Read the model definition and answer for the solid it produces. Units are mm, in the model's axes. Give positions to 0.01 mm unless a question says otherwise; leave off trailing zeros. Loops run counter-clockwise (first coordinate to the right, second up) from the corner with the lowest first, then second, coordinate; pieces in that order, holes last. Notation, with made-up numbers: (82.25, 66.25) -> (98.25, 66.25) arc R11 ccw to (98.25, 85.25) -> close; hole circle Ø8 at (87.5, 74.5). An arc over 180 degrees is marked (long way). Return JSON: item names as keys, results as strings. Group by question number.
from build123d import *

# Parameters (mm, degrees)
BOSS_EXTRUDE1_DEPTH      = 192.925743
BOSS_EXTRUDE1_DEPTH_BACK = 146.220291
SKETCH1_R                = 7.9375
SKETCH1_R_2              = 6.4643
CUT_EXTRUDE1_DEPTH       = 331.187461377


with BuildPart() as part:
    # Sketch1 → Boss-Extrude1 (new, two sides: drawn at the far end of the back side and taken through both)
    with BuildSketch(Plane(origin=(0, 0, 0), x_dir=(0, 0, -1), z_dir=(1, 0, 0)).offset(-BOSS_EXTRUDE1_DEPTH_BACK)):
        with Locations(Location((0, 0, 0), (0, 0, 180))):
            Circle(SKETCH1_R)
        with Locations(Location((0, 0, 0), (0, 0, 180))):
            Circle(SKETCH1_R_2, mode=Mode.SUBTRACT)
    extrude(amount=BOSS_EXTRUDE1_DEPTH + BOSS_EXTRUDE1_DEPTH_BACK)

    # Sketch2 → Cut-Extrude1 (cut, through all)
    with BuildSketch(Plane(origin=(179.090362215, 7.9375, -46.327801352), x_dir=(0.11485518524691138, 0, -0.9933822458761269), z_dir=(0, 1, 0))):
        with BuildLine():
            Line((-86.538819377, 317.472174359), (-82.162836819, 279.624310791))
            ThreePointArc((-82.162836819, 279.624310791), (-81.572017256, 278.562611401), (-80.403509897, 278.229649083))
            Line((-80.403509897, 278.229649083), (-77.249521267, 278.594314296))
            ThreePointArc((-77.249521267, 278.594314296), (-76.187821877, 279.185133859), (-75.854859558, 280.353641218))
            Line((-75.854859558, 280.353641218), (-80.230842116, 318.201504786))
            Line((-80.230842116, 318.201504786), (-86.538819377, 317.472174359))
        make_face()
    extrude(amount=-CUT_EXTRUDE1_DEPTH, mode=Mode.SUBTRACT)


solid = part.part
1. Section A-A on y = 0 is taken. Determine the outline of the cut face in (x, z).
2. Section B-B on x = -116.5 is taken. Determine the outline of the cut face in (y, z) (1 decimal), then the cut area to 3 significant figures.
3. Determine the mould class of faces 1 (the cylindrical face through (20.98, -6.41, -0.84)), 2 (the cylindrical face through (20.979, -2.384, 7.571)), 3 (the flat face through (192.926, 0, -7)) for opening direction Y: pulls with the +Y half, pulls with the -Y half, needs draft (parallel to the pull), parting line crosses it, or undercut.
4. Section C-C on x = 71 is taken. Determine the outline of the cut face in (y, z) (1 decimal).
5. Straight lines are drawn through the part: line 1 (Z direction, x = 152, y = -1.5); line 2 (Y direction, x = 31, z = 0.25). For each, find the intervals that lie inside material, in ascending order. Write a range as from..to.
6. Flat-ended cylindrical pins translate along their axes: pin 1 Ø1.3 at (x, y) = (-126, 6) entering from -Z; pin 2 Ø1.5 at (x, y) = (31.5, -3) entering from +Z; pin 3 Ø3 at (x, y) = (150, 4.5) entering from -Z. Find the tip coordinate at first contact, or state that the pin passes through.
Completed:
{
 "1": {"outline": "(-146.22, -7.94) -> (192.93, -7.94) -> (192.93, -6.46) -> (-146.22, -6.46) -> close; (-146.22, 6.46) -> (192.93, 6.46) -> (192.93, 7.94) -> (-146.22, 7.94) -> close"},
 "2": {"outline": "(-7.3, -3.2) arc R7.9 ccw to (7.3, -3.2) -> (5.6, -3.2) arc R6.5 cw to (-5.6, -3.2) -> close; (-7.3, 3.2) -> (-5.6, 3.2) arc R6.5 cw to (5.6, 3.2) -> (7.3, 3.2) arc R7.9 ccw to start", "area": "47.3 mm²"},
 "3": {"face 1": "undercut", "face 2": "parting line crosses it", "face 3": "needs draft"},
 "4": {"outline": "circle Ø15.9 at (0, 0); hole circle Ø12.9 at (0, 0)"},
 "5": {"line 1": "z = -7.79..-6.29, 6.29..7.79", "line 2": "y = -7.93..-6.46, 6.46..7.93"},
 "6": {"pin 1": "stops at z = -5.86", "pin 2": "stops at z = 7.61", "pin 3": "stops at z = -7.35"}
}
